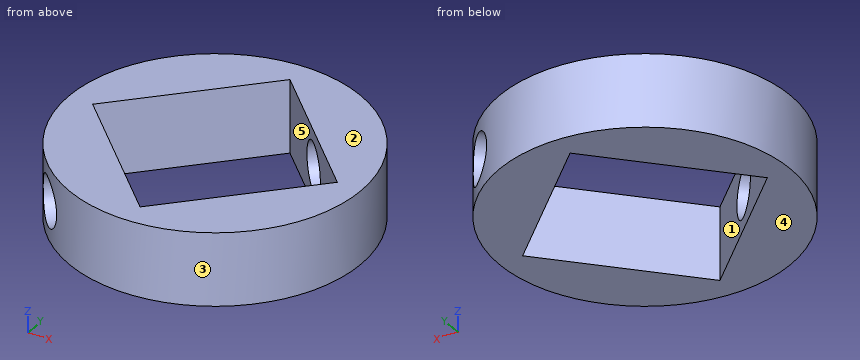
```python
from build123d import *

# Parameters (mm, degrees)
SKETCH_1_R          = 12
EXTRUDE_1_DEPTH     = 6
CUT_EXTRUDE_1_DEPTH = 10
CUT_EXTRUDE_6_DEPTH = 11
CUT_EXTRUDE_START   = -11
CUT_EXTRUDE_7_DEPTH = 11


with BuildPart() as part:
    # 草图1 → 凸台-拉伸1 (new body)
    with BuildSketch(Plane.XY):
        Circle(SKETCH_1_R)
    extrude(amount=-EXTRUDE_1_DEPTH)

    # 草图2 → 切除-拉伸1 (cut)
    with BuildSketch(Plane.XY):
        Polygon((10, 0), (0, 10), (-10, 0), (0, -10), align=None)
    extrude(amount=-CUT_EXTRUDE_1_DEPTH, mode=Mode.SUBTRACT)

    # 草图7 → 切除-拉伸6 (cut)
    with BuildSketch(Plane(origin=(5, 5, 0), x_dir=(0, 0, 1), z_dir=(-0.7071067811865477, -0.7071067811865475, 0))):
        with BuildLine():
            ThreePointArc((-1, 0), (-3, 2), (-5, 0))
            Line((-5, 0), (-1, 0))
        make_face()
        with BuildLine():
            Line((-1, 0), (-5, 0))
            ThreePointArc((-5, 0), (-3, -2), (-1, 0))
        make_face()
    extrude(amount=-CUT_EXTRUDE_6_DEPTH, mode=Mode.SUBTRACT)

    # 草图8 → 切除-拉伸7 (cut)
    with BuildSketch(Plane(origin=(-5, -5, 0), x_dir=(0, 0, -1), z_dir=(0.7071067811865477, 0.7071067811865475, 0)).offset(CUT_EXTRUDE_START)):
        with BuildLine():
            ThreePointArc((1, 0), (3, -2), (5, 0))
            Line((5, 0), (1, 0))
        make_face()
        with BuildLine():
            Line((1, 0), (5, 0))
            ThreePointArc((5, 0), (3, 2), (1, 0))
        make_face()
    extrude(amount=CUT_EXTRUDE_7_DEPTH, mode=Mode.SUBTRACT)


solid = part.part
```
Check sheet for the modelled part. Datum: model origin and axes. Units: mm. Face numbers are marked on the shaded views. A direction names the side the tool comes from. Give positions to 0.01 mm unless a question says otherwise; leave off trailing zeros. Loops run counter-clockwise (first coordinate to the right, second up) from the corner with the lowest first, then second, coordinate; pieces in that order, holes last. Notation, with made-up numbers: (-17.75, 62) - (27.25, 62) arc R12 cw to (27.25, 75) - close; hole circle Ø3 at (42, -17). An arc over 180 degrees is marked (long way). One line per question, with ' | ' between items. Start each with the question number.
1. Cross-section at D-D, the plane z = -3.75. Enter the section's corners in (x, y), plus the area to 3 significant figures.
2. Cross-section at A-A, the plane z = -2. Enter the section's corners in (x, y), plus the area to 3 significant figures.
3. Gauge pin test, flat ends, axial feed: pin 1 Ø3 at (y, z) = (9, -3) entering from +X; pin 2 Ø2 at (y, z) = (-9.5, -3.5) entering from -X; pin 3 Ø1.5 at (y, z) = (-7, -3.5) entering from +X. Record the tip position at first contact, or that the pin passes through.
4. Draft check along X on the marked faces 1, 2 and 3. Enter one of: released by +X, released by -X, zero draft, split by the parting line, or undercut.
5. Cross-section at C-C, the plane z = -5.5. Enter the section's corners in (x, y), plus the area to 3 significant figures.
6. Material ranges on line 1 along Y through (x, z) = (-9.75, -1.25); line 2 along X through (y, z) = (-6.75, -3.5); line 3 along X through (y, z) = (0.75, -0.75), recorded low to high. Write a range as [from, to].
7. Set-up check for the marked faces 4 and 5: record each of +Z, -Z, +X, -X, +Y, -Y from which the full face is reachable in a straight line by a thin tool's end or side.
8. Cross-section at B-B, the plane x = -2. Enter the section's corners in (y, z).
Check result:
1) outline: (-10, 0) - (0, 10) - (3.69, 6.31) - (7.07, 9.69) arc R12 ccw to (-9.69, -7.07) - (-6.31, -3.69) - close; (-7.07, -9.69) arc R12 ccw to (9.69, 7.07) - (6.31, 3.69) - (10, 0) - (0, -10) - (-3.69, -6.31) - close | area: 216 mm2
2) outline: (-10, 0) - (0, 10) - (3.78, 6.22) - (7.17, 9.62) arc R12 ccw to (-9.62, -7.17) - (-6.22, -3.78) - close; (-7.17, -9.62) arc R12 ccw to (9.62, 7.17) - (6.22, 3.78) - (10, 0) - (0, -10) - (-3.78, -6.22) - close | area: 219 mm2
3) pin 1: stops at x = 7.45 | pin 2: stops at x = -7.49 | pin 3: stops at x = 10.24
4) face 1: undercut | face 2: zero draft | face 3: split by the parting line
5) outline: circle Ø24 at (0, 0); hole (-10, 0) - (0, -10) - (10, 0) - (0, 10) - close | area: 252 mm2
6) line 1: y = [-7, -0.25], [0.25, 7] | line 2: x = [-9.92, -9.49], [-4.01, -3.25], [3.25, 9.92] | line 3: x = [-11.98, -9.25], [9.25, 11.98]
7) face 4: -Z, +X, -X, +Y, -Y | face 5: +Z, -Z
8) outline: (-11.83, -6) - (-8, -6) - (-8, 0) - (-11.83, 0) - close; (8, -6) - (11.83, -6) - (11.83, 0) - (8, 0) - close
